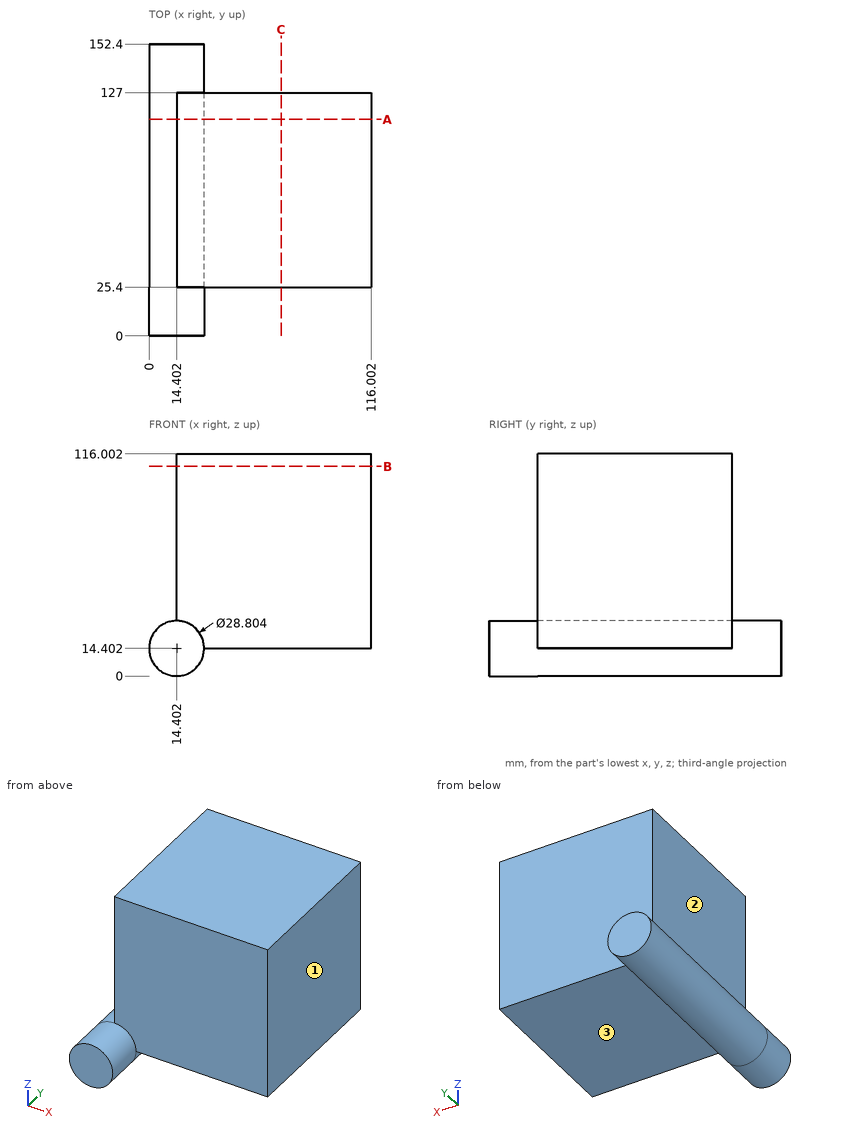
Verification items for this drawing (mm, ordinates from the low corner). A direction names the side the tool comes from. Give positions to 0.01 mm unless a question says otherwise; leave off trailing zeros. Loops run counter-clockwise (first coordinate to the right, second up) from the corner with the lowest first, then second, coordinate; pieces in that order, holes last.
(1) Thickness scan on L1, parallel to Z at x = 64.5, y = 121; L2, parallel to Y at x = 29, z = 98.5. Record the ranges inside material, lowest first.
From the geometry:
L1: z = 14.4 to 116
L2: y = 25.4 to 127
(2) Depth check by flat-ended pin: pin 1 Ø3 at (y, z) = (38.5, 81.5) entering from -X; pin 2 Ø3 at (x, z) = (99, 70.5) entering from -Y; pin 3 Ø4 at (x, z) = (67.5, 73) entering from +Y. Enter the tip coordinate at first touch or a pass-through.
From the geometry:
pin 1: stops at x = 14.4
pin 2: stops at y = 25.4
pin 3: stops at y = 127
(3) Section check A-A on y = 113. Record the cut outline in (x, z).
From the geometry:
outline: (14.4, 28.8) arc R14.4 ccw (long way) to (28.8, 14.4) - (116, 14.4) - (116, 116) - (14.4, 116) - close
(4) Section check B-B on z = 109.5. Record the cut outline in (x, y), then the cut area to 3 significant figures.
From the geometry:
outline: (14.4, 25.4) - (116, 25.4) - (116, 127) - (14.4, 127) - close
area: 10,300 mm2
(5) Section check C-C on x = 69. Record the cut outline in (y, z).
From the geometry:
outline: (25.4, 14.4) - (127, 14.4) - (127, 116) - (25.4, 116) - close
(6) Set-up check for the marked faces 1, 2 and 3: record each of +Z, -Z, +X, -X, +Y, -Y from which the full face is reachable in a straight line by a thin tool's end or side.
From the geometry:
face 1: +Z, -Z, +X, +Y, -Y
face 2: +Z, -X, +Y, -Y
face 3: -Z, +X, +Y, -Y
